For this review, take the finished solid that the model builds, in its own axes (mm). Round coordinates to 2 decimals unless told otherwise and drop trailing zeros. Order: outer loops, then holes, each group sorted by start corner. A loop starts at its lowest first (then second) coordinate and runs counter-clockwise, first axis right, second up. Notation, with made-up numbers: M -31,-28.5 L 20,-28.5 A22 cw 20,10.5 Z; hole C 34,-32.5 d10. An arc over 180 degrees is marked long. Answer as a JSON object with one key per item and string values.
from build123d import *

# Parameters (mm, degrees)
BOSS_EXTRUDE1_DEPTH = 0.5
FILLET1_R           = 0.1


with BuildPart() as part:
    # Sketch1 → Boss-Extrude1 (new body)
    with BuildSketch(Plane(origin=(0, 0, 0), x_dir=(1, 0, 0), z_dir=(0, 1, 0))):
        with BuildLine():
            Line((-7.405833782, 9.18660035), (-6.230046676, 9.685692366))
            ThreePointArc((-6.230046676, 9.685692366), (-5.641408049, 9.216396236), (-4.892259398, 9.29062958))
            ThreePointArc((-4.892259398, 9.29062958), (3.847452899, 9.769703485), (9.913592586, 3.459867344))
            ThreePointArc((9.913592586, 3.459867344), (10.597684768, 2.354472244), (11.685163211, 1.642242591))
            ThreePointArc((11.685163211, 1.642242591), (2.904608858, -11.436924735), (-11.052731833, -4.132447099))
            ThreePointArc((-11.052731833, -4.132447099), (-11.381077163, 3.116261), (-7.405833782, 9.18660035))
        make_face()
        with BuildLine():
            Line((-1.5, 6.5), (1.5, 6.5))
            Line((1.5, 6.5), (1.5, 7.858116823))
            ThreePointArc((1.5, 7.858116823), (0, -8), (-1.5, 7.858116823))
            Line((-1.5, 7.858116823), (-1.5, 6.5))
        make_face(mode=Mode.SUBTRACT)
    extrude(amount=BOSS_EXTRUDE1_DEPTH)

    # Fillet1
    fillet1_edges = [part.edges().sort_by_distance(p)[0] for p in [
        (-1.5, 0.25, -7.858116823),
        (1.5, 0.25, -7.858116823),
    ]]
    fillet(fillet1_edges, radius=FILLET1_R)


solid = part.part
1) Mouldability with a two-part tool opening along Z and no side actions: class faces 1 (the flat face through (-2, 0.5, 8)), 2 (the cylindrical face through (3.73, 0.246, -9.815)), 3 (the cylindrical face through (0.329, 0.246, 7.993)) as +Z half, -Z half, draft (parallel to the pull), parting line (faces both ways), or undercut.
Geometry check:
{"face 1": "draft", "face 2": "-Z half", "face 3": "undercut"}
2) Add section C-C on y = 0.4. State the section outline as (x, z) points, and give its area (3 significant figures).
Geometry check:
{"outline": "M -7.41,-9.19 L -6.23,-9.69 A1 cw -4.89,-9.29 A10.5 ccw 9.91,-3.46 A3 cw 11.69,-1.64 A11.8 ccw long Z; hole M -1.62,-7.83 A0.1 ccw -1.5,-7.74 L -1.5,-6.5 L 1.5,-6.5 L 1.5,-7.74 A0.1 ccw 1.62,-7.83 A8 ccw long Z", "area": "212 mm²"}
3) Insertion check: P1, Ø8, axis at x = -2.5, z = -2, coming from the +Y side. The pin has a flat end and moves straight along its axis. Give the tip position at first contact, or say it passes through.
Geometry check:
{"P1": "passes through"}
4) Add section A-A on z = 0. State the section outline as (x, y) points, and give its area (3 significant figures).
Geometry check:
{"outline": "M -11.8,0 L -8,0 L -8,0.5 L -11.8,0.5 Z; M 8,0 L 11.8,0 L 11.8,0.5 L 8,0.5 Z", "area": "3.80 mm²"}
5) For L1, parallel to X at y = 0.2, z = 0; L2, parallel to X at y = 0.15, z = -3; L3, parallel to Z at x = -0.75, y = 0.15, list the stretches that pass through material, from the lowest coordinate up.
Geometry check:
{"L1": "x = -11.8 to -8, 8 to 11.8", "L2": "x = -11.41 to -7.42, 7.42 to 10.12", "L3": "z = -10.47 to -6.5, 7.96 to 11.78"}
6) Add section D-D on z = -8.25. State the section outline as (x, y) points.
Geometry check:
{"outline": "M -8.44,0 L 6.5,0 L 6.5,0.5 L -8.44,0.5 Z"}
7) Add section B-B on x = 0. State the section outline as (y, z) points.
Geometry check:
{"outline": "M 0,-10.5 L 0.5,-10.5 L 0.5,-6.5 L 0,-6.5 Z; M 0,8 L 0.5,8 L 0.5,11.8 L 0,11.8 Z"}
